from build123d import *

# Parameters (mm, degrees)
SKETCH_1_R          = 25
EXTRUDE_1_DEPTH     = 8.5
SKETCH_2_R          = 22.05
CUT_EXTRUDE_1_DEPTH = 6.1
SKETCH_3_R          = 18.05
CUT_EXTRUDE_2_DEPTH = 12.5
FILLET_2_R          = 2
EXTRUDE_3_DEPTH     = 8.5
SKETCH_8_R          = 3.2
SKETCH_8_R_2        = 1.6
CUT_EXTRUDE_3_DEPTH = 2
SKETCH_8_2_R        = 1.6
CUT_EXTRUDE_4_DEPTH = 10
FILLET_3_R          = 4
CUT_EXTRUDE_5_DEPTH = 10
FILLET_5_R          = 8
FILLET_6_R          = 20


with BuildPart() as part:
    # Sketch 1 → Extrude 1 (new body)
    with BuildSketch(Plane(origin=(0, 0, 0), x_dir=(1, 0, 0), z_dir=(0, 1, 0))):
        with Locations(Location((0, 0, 0), (0, 0, 270))):
            Circle(SKETCH_1_R)
    extrude(amount=EXTRUDE_1_DEPTH)

    # Sketch 2 → Cut-Extrude 1 (cut)
    with BuildSketch(Plane(origin=(0, 8.5, 0), x_dir=(1, 0, 0), z_dir=(0, 1, 0))):
        with Locations(Location((0, 0, 0), (0, 0, 270))):
            Circle(SKETCH_2_R)
    extrude(amount=-CUT_EXTRUDE_1_DEPTH, mode=Mode.SUBTRACT)

    # Sketch 3 → Cut-Extrude 2 (cut)
    with BuildSketch(Plane(origin=(0, 2.4, 0), x_dir=(1, 0, 0), z_dir=(0, 1, 0))):
        with Locations(Location((0, 0, 0), (0, 0, 270))):
            Circle(SKETCH_3_R)
    extrude(amount=-CUT_EXTRUDE_2_DEPTH, mode=Mode.SUBTRACT)

    # Fillet 2
    fillet_2_edges = [part.edges().sort_by_distance(p)[0] for p in [
        (0, 8.5, -22.05),
    ]]
    fillet(fillet_2_edges, radius=FILLET_2_R)

    # Sketch 7 → Extrude 3 (add)
    with BuildSketch(Plane.XZ):
        with BuildLine():
            ThreePointArc((-25, -4.2e-08), (-17.677669545, 17.677669515), (0, 25))
            Line((0, 25), (-25, 25))
            Line((-25, 25), (-25, -4.2e-08))
        make_face()
        with BuildLine():
            Line((25, 25), (0, 25))
            ThreePointArc((0, 25), (17.67766953, 17.67766953), (25, 0))
            Line((25, 0), (25, 25))
        make_face()
        with BuildLine():
            ThreePointArc((25, 0), (17.67766953, -17.67766953), (0, -25))
            Line((0, -25), (0, -29))
            Line((0, -29), (25, -29))
            Line((25, -29), (25, 0))
        make_face()
        with BuildLine():
            Line((0, -29), (0, -25))
            ThreePointArc((0, -25), (-17.677669515, -17.677669545), (-25, -4.2e-08))
            Line((-25, -4.2e-08), (-25, -29))
            Line((-25, -29), (0, -29))
        make_face()
    extrude(amount=-EXTRUDE_3_DEPTH)

    # Sketch 8 → Cut-Extrude 3 (cut)
    # profile 1 of 4: a face of its own
    with BuildSketch(Plane.XZ):
        with Locations(Location((-20, 15, 0), (0, 0, 270))):
            Circle(SKETCH_8_R)
        with Locations(Location((-20, 15, 0), (0, 0, 270))):
            Circle(SKETCH_8_R_2, mode=Mode.SUBTRACT)
    # profile 2 of 4: a face of its own
    with BuildSketch(Plane.XZ):
        with Locations(Location((20, 15, 0), (0, 0, 270))):
            Circle(SKETCH_8_R)
        with Locations(Location((20, 15, 0), (0, 0, 270))):
            Circle(SKETCH_8_R_2, mode=Mode.SUBTRACT)
    # profile 3 of 4: a face of its own
    with BuildSketch(Plane.XZ):
        with Locations(Location((20, -25, 0), (0, 0, 270))):
            Circle(SKETCH_8_R)
        with Locations(Location((20, -25, 0), (0, 0, 270))):
            Circle(SKETCH_8_R_2, mode=Mode.SUBTRACT)
    # profile 4 of 4: a face of its own
    with BuildSketch(Plane.XZ):
        with Locations(Location((-20, -25, 0), (0, 0, 270))):
            Circle(SKETCH_8_R)
        with Locations(Location((-20, -25, 0), (0, 0, 270))):
            Circle(SKETCH_8_R_2, mode=Mode.SUBTRACT)
    extrude(amount=-CUT_EXTRUDE_3_DEPTH, mode=Mode.SUBTRACT)

    # Sketch 8_2 → Cut-Extrude 4 (cut)
    with BuildSketch(Plane.XZ):
        with Locations(Location((-20, 15, 0), (0, 0, 270))):
            Circle(SKETCH_8_2_R)
        with Locations(Location((20, 15, 0), (0, 0, 270))):
            Circle(SKETCH_8_2_R)
        with Locations(Location((20, -25, 0), (0, 0, 270))):
            Circle(SKETCH_8_2_R)
        with Locations(Location((-20, -25, 0), (0, 0, 270))):
            Circle(SKETCH_8_2_R)
    extrude(amount=-CUT_EXTRUDE_4_DEPTH, mode=Mode.SUBTRACT)

    # Fillet 3
    fillet_3_edges = [part.edges().sort_by_distance(p)[0] for p in [
        (25, 4.25, -29),
        (-25, 4.25, -29),
    ]]
    fillet(fillet_3_edges, radius=FILLET_3_R)

    # Sketch 9 → Cut-Extrude 5 (cut)
    with BuildSketch(Plane.XZ):
        with BuildLine():
            Line((-25, 25), (-25, 16.656703877))
            ThreePointArc((-25, 16.656703877), (-19.906442689, 21.414889027), (-13.928848582, 25))
            Line((-13.928848582, 25), (-25, 25))
        make_face()
        with BuildLine():
            Line((25, 25), (13.928848582, 25))
            ThreePointArc((13.928848582, 25), (19.906442689, 21.414889027), (25, 16.656703877))
            Line((25, 16.656703877), (25, 25))
        make_face()
    extrude(amount=-CUT_EXTRUDE_5_DEPTH, mode=Mode.SUBTRACT)

    # Fillet 5
    fillet_5_edges = [part.edges().sort_by_distance(p)[0] for p in [
        (-25, 4.25, 16.656703877),
        (25, 4.25, 16.656703877),
    ]]
    fillet(fillet_5_edges, radius=FILLET_5_R)

    # Fillet 6
    fillet_6_edges = [part.edges().sort_by_distance(p)[0] for p in [
        (-13.928848582, 4.25, 25),
        (13.928848582, 4.25, 25),
    ]]
    fillet(fillet_6_edges, radius=FILLET_6_R)


solid = part.part
Model file for the job. Use its own axes, mm. A direction names the side the tool comes from. Give positions to 0.01 mm unless a question says otherwise; leave off trailing zeros. Loops run counter-clockwise (first coordinate to the right, second up) from the corner with the lowest first, then second, coordinate; pieces in that order, holes last. Notation, with made-up numbers: (-25.75, -34.75) -> (26.25, -34.75) arc R23 cw to (26.25, -22.75) -> close; hole circle Ø8 at (-39, 55.5). An arc over 180 degrees is marked (long way). Use a Markdown table: item, result. Add a question column.
(1) Tool access for faces 1 (the cylindrical face through (-24.346, 4.31, 16.601)), 2 (the cylindrical face through (-13.417, 4.479, -17.498)), 3 (the flat face through (18.6, 2, -26.4)): list every direction of +Z, -Z, +X, -X, +Y, -Y with a clear straight run to the whole face (end or side of a thin tool).
(2) Slice it at A-A on z = 0. List the corners of the cut face in (x, y), and give its area (3 significant figures).
(3) Drop flat-ended pins along their axis: pin 1 Ø4 at (x, z) = (-20, 15) entering from -Y; pin 2 Ø10 at (x, z) = (-14, 0.5) entering from +Y. Give the stop position or say it passes through.
(4) Wall check: line 1 along X through (y, z) = (3, -25.5); line 2 along X through (y, z) = (5.1, 0); line 3 along X through (y, z) = (2.25, -0.5). Give the ranges that are in metal, low to high.
(5) Slice it at B-B on y = 5.5. List the corners of the cut face in (x, z).
(6) Mould opens along Z. For faces 4 (the flat face through (25, 4, -6)), 5 (the cylindrical face through (-21.881, 4.19, 19.804)), 6 (the cylindrical face through (-18.414, 5.204, -24.792)) say: +Z half, -Z half, draft (parallel to the pull), parting line (faces both ways), or undercut.
Filled sheet:
| question | item | result |
|---|---|---|
| 1 | face 1 | +Z, -X, +Y, -Y |
| 1 | face 2 | +Y |
| 1 | face 3 | -Y |
| 2 | outline | (-25, 0) -> (-18.05, 0) -> (-18.05, 2.4) -> (-22.05, 2.4) -> (-22.05, 6.5) arc R2 ccw to (-24.05, 8.5) -> (-25, 8.5) -> close; (18.05, 0) -> (25, 0) -> (25, 8.5) -> (24.05, 8.5) arc R2 ccw to (22.05, 6.5) -> (22.05, 2.4) -> (18.05, 2.4) -> close |
| 2 | area | 67.6 mm2 |
| 3 | pin 1 | y = 2 |
| 3 | pin 2 | y = 2.4 |
| 4 | line 1 | -24.97 to -21.52, -18.48 to 18.48, 21.52 to 24.97 |
| 4 | line 2 | -25 to -22.05, 22.05 to 25 |
| 4 | line 3 | -25 to -18.04, 18.04 to 25 |
| 5 | outline | (-25, -25) arc R4 ccw to (-21, -29) -> (21, -29) arc R4 ccw to (25, -25) -> (25, 13.43) arc R8 ccw to (22.42, 19.31) arc R33.08 ccw to (21.31, 20.3) arc R20 ccw to (8.42, 25) -> (-8.42, 25) arc R20 ccw to (-21.31, 20.3) arc R33.08 ccw to (-22.42, 19.31) arc R8 ccw to (-25, 13.43) -> close; hole circle Ø44.1 at (0, 0); hole circle Ø3.2 at (-20, -25); hole circle Ø3.2 at (-20, 15); hole circle Ø3.2 at (20, -25); hole circle Ø3.2 at (20, 15) |
| 6 | face 4 | draft |
| 6 | face 5 | +Z half |
| 6 | face 6 | undercut |
